```python
from build123d import *

# Parameters (mm, degrees)
SKETCH1_R           = 2
BOSS_EXTRUDE1_DEPTH = 47
SKETCH2_R           = 1.5
BOSS_EXTRUDE2_DEPTH = 6.6
BOSS_EXTRUDE3_START = 6.6
SKETCH3_R           = 1.5
BOSS_EXTRUDE3_DEPTH = 6.6
CHAMFER1_SIZE       = 0.4


with BuildPart() as part:
    # Sketch1 → Boss-Extrude1 (new body)
    with BuildSketch(Plane.XY):
        Circle(SKETCH1_R)
    extrude(amount=-BOSS_EXTRUDE1_DEPTH)

    # Sketch2 → Boss-Extrude2 (add)
    with BuildSketch(Plane.XY):
        Circle(SKETCH2_R)
    extrude(amount=BOSS_EXTRUDE2_DEPTH)

    # Sketch3 → Boss-Extrude3 (add)
    with BuildSketch(Plane(origin=(0, 0, -47), x_dir=(-1, 0, 0), z_dir=(0, 0, -1)).offset(BOSS_EXTRUDE3_START)):
        with Locations(Location((0, 0, 0), (0, 0, 180))):
            Circle(SKETCH3_R)
    extrude(amount=-BOSS_EXTRUDE3_DEPTH)

    # Chamfer1
    chamfer1_edges = [part.edges().sort_by_distance(p)[0] for p in [
        (-1.5, 0, -53.6),
        (-1.5, 0, 6.6),
    ]]
    chamfer(chamfer1_edges, length=CHAMFER1_SIZE)


solid = part.part
```
Source: CAD feature listing. Evaluate the final solid. Frame: model axes, mm. A direction names the side the tool comes from. Round coordinates to 2 decimals unless told otherwise and drop trailing zeros. Loops run counter-clockwise (first coordinate to the right, second up) from the corner with the lowest first, then second, coordinate; pieces in that order, holes last.
1. Section query A-A on x = 0. Output: boundary loops of the cut face in (y, z).
2. Ray query, L1, parallel to X at y = -0.15, z = -15.5; L2, parallel to Z at x = -0.05, y = 1.8. Return the intervals inside material, ascending.
3. Section query C-C on z = -33. Output: boundary loops of the cut face in (x, y), and give its area (3 significant figures).
4. Access query for faces 1 (the flat face through (0, 0, 6.6)), 2 (the cylindrical face through (1.43, -0.45, -50.14)), 3 (the cylindrical face through (-1.5, 0.07, 3.06)). Directions: +Z, -Z, +X, -X, +Y, -Y. A direction counts if a zero-diameter tool reaches every point of the face in a straight line with its end or side. Return the directions, or none.
Answers below:
1. outline: (-2, -47) - (-1.5, -47) - (-1.5, -53.2) - (-1.1, -53.6) - (1.1, -53.6) - (1.5, -53.2) - (1.5, -47) - (2, -47) - (2, 0) - (1.5, 0) - (1.5, 6.2) - (1.1, 6.6) - (-1.1, 6.6) - (-1.5, 6.2) - (-1.5, 0) - (-2, 0) - close
2. L1: x = -1.99 to 1.99
2. L2: z = -47 to 0
3. outline: circle Ø4 at (0, 0)
3. area: 12.6 mm2
4. face 1: +Z, +X, -X, +Y, -Y
4. face 2: -Z
4. face 3: +Z
